from build123d import *

# Parameters (mm, degrees)
BOSS_EXTRUDE1_DEPTH = 0.9


with BuildPart() as part:
    # Sketch1 → Boss-Extrude1 (new body)
    with BuildSketch(Plane(origin=(0, 0, 0), x_dir=(1, 0, 0), z_dir=(0, 1, 0))):
        with BuildLine():
            Line((4.9, 4.05), (2.615181585, 4.026685526))
            Line((2.615181585, 4.026685526), (2.615181585, 3.026685526))
            ThreePointArc((2.615181585, 3.026685526), (4, 0), (2.615181585, -3.026685526))
            Line((2.615181585, -3.026685526), (2.615181585, -4.026685526))
            Line((2.615181585, -4.026685526), (4.9, -4.05))
            Line((4.9, -4.05), (4.9, 4.05))
        make_face()
    extrude(amount=BOSS_EXTRUDE1_DEPTH)


solid = part.part
Read the model definition and answer for the solid it produces. Units are mm, in the model's axes. Coordinates: 2 decimals unless noted, no trailing zeros. Loops run counter-clockwise (first coordinate to the right, second up) from the corner with the lowest first, then second, coordinate; pieces in that order, holes last. Notation, with made-up numbers: (-22.5, 8) -> (16.5, 8) arc R29 cw to (16.5, 29) -> close; hole circle Ø9 at (-16, 72). An arc over 180 degrees is marked (long way). Answer in a Markdown table with one row per item.
Item 1: For a pull along Z with two mould halves and no side action, classify faces 1 (the flat face through (4.2, 0.9, -0.1)), 2 (the cylindrical face through (4, 0.4, 0)) as released by +Z, released by -Z, zero draft, split by the parting line, or undercut.
Returned:
| item | result |
|---|---|
| face 1 | zero draft |
| face 2 | undercut |
Item 2: A cutting plane is placed at B-B on y = 0.1. Determine the outline of the cut face in (x, z).
Returned:
| item | result |
|---|---|
| outline | (2.62, -4.03) -> (4.9, -4.05) -> (4.9, 4.05) -> (2.62, 4.03) -> (2.62, 3.03) arc R4 cw to (2.62, -3.03) -> close |
Item 3: A cutting plane is placed at D-D on z = 0.25. Determine the outline of the cut face in (x, y), plus the area to 3 significant figures.
Returned:
| item | result |
|---|---|
| outline | (3.99, 0) -> (4.9, 0) -> (4.9, 0.9) -> (3.99, 0.9) -> close |
| area | 0.817 mm^2 |
Item 4: A cutting plane is placed at A-A on x = 3.05. Determine the outline of the cut face in (y, z).
Returned:
| item | result |
|---|---|
| outline | (0, -4.03) -> (0.9, -4.03) -> (0.9, -2.59) -> (0, -2.59) -> close; (0, 2.59) -> (0.9, 2.59) -> (0.9, 4.03) -> (0, 4.03) -> close |
Item 5: Straight lines are drawn through the part: line 1 along Z through (x, y) = (3.1, 0.7); line 2 along Z through (x, y) = (3, 0.6); line 3 along Z through (x, y) = (4.65, 0.55). For each, find the intervals that lie inside material, in ascending order. Write a range as [from, to].
Returned:
| item | result |
|---|---|
| line 1 | z = [-4.03, -2.53], [2.53, 4.03] |
| line 2 | z = [-4.03, -2.65], [2.65, 4.03] |
| line 3 | z = [-4.05, 4.05] |
Item 6: A cutting plane is placed at C-C on x = 3.5. Determine the outline of the cut face in (y, z).
Returned:
| item | result |
|---|---|
| outline | (0, -4.04) -> (0.9, -4.04) -> (0.9, -1.94) -> (0, -1.94) -> close; (0, 1.94) -> (0.9, 1.94) -> (0.9, 4.04) -> (0, 4.04) -> close |
